Geometry: final body of the model. Coordinates: model frame, mm. Face numbers are marked on the shaded views. A direction names the side the tool comes from. Round coordinates to 2 decimals unless told otherwise and drop trailing zeros. Write each loop counter-clockwise with the first axis right and the second up, starting at its lowest first coordinate (ties: lowest second). Pieces come first, ordered by that corner, then holes. Notation, with made-up numbers: M 72.5,-34 L 103.5,-34 A11 ccw 103.5,-26 Z; hole C -37,74.25 d9. An arc over 180 degrees is marked long. Use one line per item in the form item = value. Start each with the question number.
Item 1: Section query D-D (x = 66). Return loops of the section in (y, z), and give its area (3 significant figures).
Item 2: Reachability of the marked faces 1, 2 and 3 from +Z, -Z, +X, -X, +Y, -Y: full face, straight path, thin tool, end or side. Return the list, or none.
Item 3: Section query B-B (y = 45). Return loops of the section in (x, z), and give its area (3 significant figures).
Item 4: Pin query (flat end, axial travel): pin 1 Ø4 at (x, y) = (85.25, -5) entering from +Z; pin 2 Ø0.6 at (y, z) = (34.5, 3) entering from -X; pin 3 Ø2.5 at (y, z) = (44.5, 5) entering from -X. Return the tip coordinate at first contact, or that it passes through.
Item 5: Section query A-A (z = 6.75). Return loops of the section in (x, y).
Item 6: Pull-direction query (Y, two-part tool) for the marked faces 4, 5 and 6; classes: pulls with the +Y half, pulls with the -Y half, needs draft (parallel to the pull), parting line crosses it, or undercut.
Item 7: Section query C-C (x = -5). Return loops of the section in (y, z).
Item 8: Ray query, probe 1 along Y at (x, z) = (85.25, 6.7); probe 2 along Y at (x, z) = (86, 6.75); probe 3 along Z at (x, y) = (17.5, 22). Return the intervals inside material, ascending.
from build123d import *

# Parameters (mm, degrees)
PAD_DEPTH       = 2
SKETCH017_W     = 10
SKETCH017_H     = 9.5
SKETCH017_W_2   = 9.5
SKETCH017_H_2   = 10
PAD006_DEPTH    = 2
SKETCH018_W     = 10
SKETCH018_H     = 9.5
SKETCH018_W_2   = 9.5
SKETCH018_H_2   = 10
PAD007_DEPTH    = 10
SKETCH020_R     = 1.6
POCKET008_DEPTH = 9
POCKET011_DEPTH = 4
FILLET002_R     = 2
SKETCH028_W     = 3
SKETCH028_H     = 2
PAD010_DEPTH    = 3
CHAMFER_SIZE    = 2


with BuildPart() as part:
    # Sketch → Pad (new body)
    with BuildSketch(Plane.XY):
        with BuildLine():
            Line((5, 0), (90, 0))
            ThreePointArc((90, 0), (93.5355339059, 1.4644660941), (95, 5))
            Line((95, 5), (95, 35))
            ThreePointArc((95, 35), (93.5355339059, 38.5355339059), (90, 40))
            Line((90, 40), (5, 40))
            ThreePointArc((5, 40), (1.4644660941, 38.5355339059), (0, 35))
            Line((0, 35), (0, 5))
            ThreePointArc((0, 5), (1.4644660941, 1.4644660941), (5, 0))
        make_face()
    extrude(amount=PAD_DEPTH)

    # Sketch017 (on Face10 of Pad) → Pad006 (join)
    with BuildSketch(Plane.XY.offset(2)):
        with Locations((-5, 21.75)):
            Rectangle(SKETCH017_W, SKETCH017_H)
        with Locations((85.25, -5)):
            Rectangle(SKETCH017_W_2, SKETCH017_H_2)
        with Locations((85.25, 45)):
            Rectangle(SKETCH017_W_2, SKETCH017_H_2)
    extrude(amount=-PAD006_DEPTH)

    # Sketch018 (on Face18 of Pad006) → Pad007 (join)
    with BuildSketch(Plane.XY.offset(2)):
        with Locations((-5, 21.75)):
            Rectangle(SKETCH018_W, SKETCH018_H)
        with Locations((85.25, -5)):
            Rectangle(SKETCH018_W_2, SKETCH018_H_2)
        with Locations((85.25, 45)):
            Rectangle(SKETCH018_W_2, SKETCH018_H_2)
    extrude(amount=PAD007_DEPTH)

    # Sketch020 (on Face29 of Pad007) → Pocket008 (cut)
    with BuildSketch(Plane.XY.offset(12)):
        with Locations((85.25, -5)):
            Circle(SKETCH020_R)
        with Locations((85.25, 45)):
            Circle(SKETCH020_R)
        with Locations((-5, 21.75)):
            Circle(SKETCH020_R)
    extrude(amount=-POCKET008_DEPTH, mode=Mode.SUBTRACT)

    # Sketch021 (on Face29 of Pocket008) → Pocket011 (cut)
    with BuildSketch(Plane.XY.offset(12)):
        Polygon((87.9346787517, 43.45), (87.9346787517, 46.55), (85.25, 48.1), (82.5653212483, 46.55), (82.5653212483, 43.45), (85.25, 41.9), align=None)
        Polygon((87.9346787517, -6.55), (87.9346787517, -3.45), (85.25, -1.9), (82.5653212483, -3.45), (82.5653212483, -6.55), (85.25, -8.1), align=None)
        Polygon((-3.45, 19.0653212483), (-1.9, 21.75), (-3.45, 24.4346787517), (-6.55, 24.4346787517), (-8.1, 21.75), (-6.55, 19.0653212483), align=None)
    extrude(amount=-POCKET011_DEPTH, mode=Mode.SUBTRACT)

    # Fillet002
    fillet002_edges = [part.edges().sort_by_distance(p)[0] for p in [
        (-10, 17, 7),
        (-10, 26.5, 7),
        (80.5, 50, 7),
        (90, 50, 7),
        (80.5, -10, 7),
        (90, -10, 7),
    ]]
    fillet(fillet002_edges, radius=FILLET002_R)

    # Sketch028 (on Face12 of Fillet002) → Pad010 (join)
    with BuildSketch(Plane.XY.offset(2)):
        with Locations((73.5, 34)):
            Rectangle(SKETCH028_W, SKETCH028_H)
        with Locations((73.5, 6)):
            Rectangle(SKETCH028_W, SKETCH028_H)
    extrude(amount=PAD010_DEPTH)

    # Chamfer
    chamfer_edges = [part.edges().sort_by_distance(p)[0] for p in [
        (75, 6, 5),
        (75, 34, 5),
    ]]
    chamfer(chamfer_edges, length=CHAMFER_SIZE)


solid = part.part
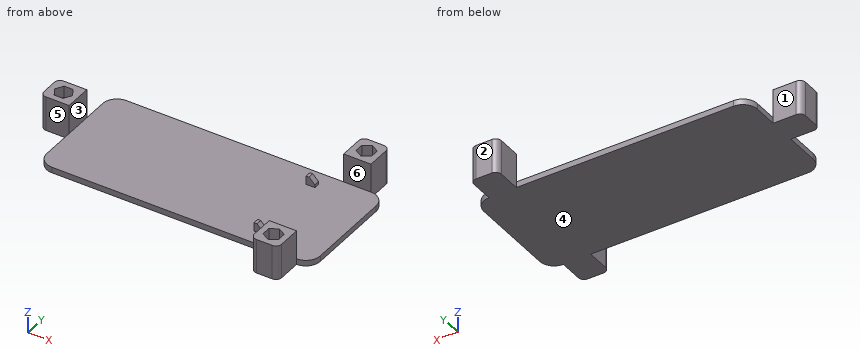
Working result:
q1.outline = M 0,0 L 40,0 L 40,2 L 0,2 Z
q1.area = 80.0 mm²
q2.face_1 = +Z, -Z, -X, +Y
q2.face_2 = +Z, -Z, +X, -X, +Y
q2.face_3 = +Z, +X, +Y, -Y
q3.outline = M 80.5,0 L 90,0 L 90,12 L 87.93,12 L 87.93,8 L 86.85,8 L 86.85,3 L 83.65,3 L 83.65,8 L 82.57,8 L 82.57,12 L 80.5,12 Z
q3.area = 76.5 mm²
q4.pin_1 = 8
q4.pin_2 = 72
q4.pin_3 = 80.5
q5.outline = M -10,19 A2 ccw -8,17 L 0,17 L 0,26.5 L -8,26.5 A2 ccw -10,24.5 Z; M 80.5,-8 A2 ccw 82.5,-10 L 88,-10 A2 ccw 90,-8 L 90,0 L 80.5,0 Z; M 80.5,40 L 90,40 L 90,48 A2 ccw 88,50 L 82.5,50 A2 ccw 80.5,48 Z; hole C -5,21.75 d3.2; hole C 85.25,-5 d3.2; hole C 85.25,45 d3.2
q6.face_4 = needs draft
q6.face_5 = pulls with the -Y half
q6.face_6 = undercut
q7.outline = M 17,0 L 26.5,0 L 26.5,12 L 24.43,12 L 24.43,8 L 23.35,8 L 23.35,3 L 20.15,3 L 20.15,8 L 19.07,8 L 19.07,12 L 17,12 Z
q8.probe_1 = -10 to -6.6, -3.4 to 0, 40 to 43.4, 46.6 to 50
q8.probe_2 = -10 to -6.41, -3.59 to 0, 40 to 43.59, 46.41 to 50
q8.probe_3 = 0 to 2
